Source: CAD feature listing. Evaluate the final solid. Frame: model axes, mm. A direction names the side the tool comes from. Give positions to 0.01 mm unless a question says otherwise; leave off trailing zeros. Write each loop counter-clockwise with the first axis right and the second up, starting at its lowest first coordinate (ties: lowest second). Pieces come first, ordered by that corner, then holes. Notation, with made-up numbers: (-24, 43.25) -> (15, 43.25) arc R26 ccw to (15, 81.25) -> close; hole circle Ø1 at (-35.75, 65). An arc over 180 degrees is marked (long way). Answer as a JSON object with one key per item and string values. Group by question number.
Item 1: Access query for faces 5 (the face through (30.5, -10, 2.6)), 6 (the face through (13, -5, 8)), 7 (the face through (28, -5, 3)), 8 (the face through (55, -5, 14)), 9 (the face through (1, -5, 14)). Directions: +Z, -Z, +X, -X, +Y, -Y. A direction counts if a zero-diameter tool reaches every point of the face in a straight line with its end or side. Return the directions, or none.
Item 2: Section query D-D on x = 48. Return the cut outline in (y, z), plus the area to 3 significant figures.
Item 3: Pull-direction query (X, two-part tool) for faces 1 (the face through (57, -5, 17)), 2 (the face through (30.5, 0, 2.6)), 3 (the face through (8, -5, 17)), 4 (the face through (0, -5, 17)); classes: pulls with the +X half, pulls with the -X half, needs draft (parallel to the pull), parting line crosses it, or undercut.
Item 4: Section query B-B on z = 14.5. Return the cut outline in (x, y).
Item 5: First-contact query: pin 1 Ø5 at (y, z) = (-1.5, 9.5) entering from +X; pin 2 Ø2.5 at (x, y) = (1, -5) entering from -Z; pin 3 Ø3 at (x, y) = (49.5, -2.5) entering from -Z; pin 4 Ø12 at (x, z) = (27.5, 9.5) entering from +Y. Flat tips, straight axial feed; report the tip coordinate or a pass-through.
Item 6: Ray query, probe 1 along X at (y, z) = (-6, 10); probe 2 along X at (y, z) = (-4, 1.75); probe 3 along Z at (x, y) = (53, -2.5). Return the intervals inside material, ascending. Write a range as from..to.
Item 7: Section query C-C on y = -7. Return the cut outline in (x, z).
Item 8: Section query A-A on z = 10.5. Return the cut outline in (x, y), plus the area to 3 significant figures.
from build123d import *

# Parameters (mm, degrees)
SKETCH_W      = 57
SKETCH_H      = 20
PAD_DEPTH     = 10
SKETCH001_W   = 10
SKETCH001_H   = 17
SKETCH001_W_2 = 3
SKETCH001_H_2 = 14
SKETCH001_W_3 = 25
POCKET_DEPTH  = 10


with BuildPart() as part:
    # Sketch → Pad (new body)
    with BuildSketch(Plane.XZ):
        with Locations((28.5, 10)):
            Rectangle(SKETCH_W, SKETCH_H)
    extrude(amount=PAD_DEPTH)

    # Sketch001 (on Face6 of Pad) → Pocket (cut)
    with BuildSketch(Plane.XZ.offset(10)):
        with Locations((8, 8.5)):
            Rectangle(SKETCH001_W, SKETCH001_H)
        with Locations((1.5, 7)):
            Rectangle(SKETCH001_W_2, SKETCH001_H_2)
        with Locations((28.5, 11.5)):
            Rectangle(SKETCH001_W_3, SKETCH001_H)
        with Locations((49, 8.5)):
            Rectangle(SKETCH001_W, SKETCH001_H)
        with Locations((55.5, 7)):
            Rectangle(SKETCH001_W_2, SKETCH001_H_2)
    extrude(amount=-POCKET_DEPTH, mode=Mode.SUBTRACT)


solid = part.part
Worked answers:
{
 "1": {"face 5": "+Z, -Z, +X, -X, -Y", "face 6": "-Z, +Y, -Y", "face 7": "+Z, +Y, -Y", "face 8": "-Z, +X, +Y, -Y", "face 9": "-Z, -X, +Y, -Y"},
 "2": {"outline": "(-10, 17) -> (0, 17) -> (0, 20) -> (-10, 20) -> close", "area": "30.0 mm^2"},
 "3": {"face 1": "pulls with the +X half", "face 2": "needs draft", "face 3": "undercut", "face 4": "pulls with the -X half"},
 "4": {"outline": "(0, -10) -> (3, -10) -> (3, 0) -> (0, 0) -> close; (13, -10) -> (16, -10) -> (16, 0) -> (13, 0) -> close; (41, -10) -> (44, -10) -> (44, 0) -> (41, 0) -> close; (54, -10) -> (57, -10) -> (57, 0) -> (54, 0) -> close"},
 "5": {"pin 1": "x = 44", "pin 2": "z = 14", "pin 3": "z = 17", "pin 4": "through"},
 "6": {"probe 1": "13..16, 41..44", "probe 2": "13..44", "probe 3": "17..20"},
 "7": {"outline": "(0, 14) -> (3, 14) -> (3, 17) -> (13, 17) -> (13, 0) -> (44, 0) -> (44, 17) -> (54, 17) -> (54, 14) -> (57, 14) -> (57, 20) -> (41, 20) -> (41, 3) -> (16, 3) -> (16, 20) -> (0, 20) -> close"},
 "8": {"outline": "(13, -10) -> (16, -10) -> (16, 0) -> (13, 0) -> close; (41, -10) -> (44, -10) -> (44, 0) -> (41, 0) -> close", "area": "60.0 mm^2"}
}
